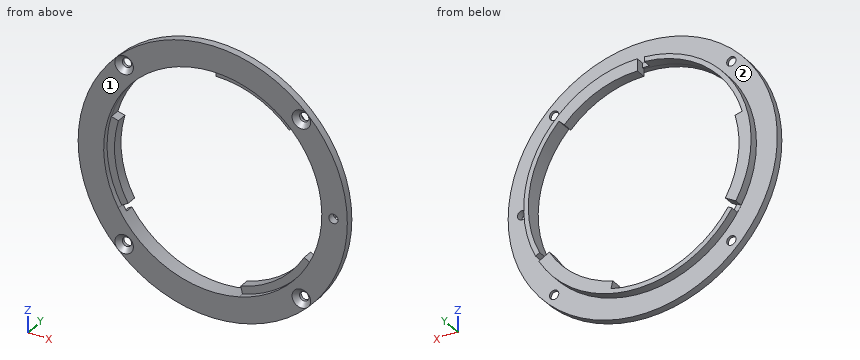
```python
from build123d import *

# Parameters (mm, degrees)
F0_R            = 29
F0_R_2          = 21.9
F1_DEPTH        = 3.5
F2_R            = 23.5
F3_DEPTH        = 1.2
F5_DEPTH        = 3.501
F6_R            = 30.5
F6_R_2          = 24.5
F7_DEPTH        = 1.9
F8_W            = 1.5
F8_H            = 25
F9_DEPTH        = 1.85
F11_D           = 2
F13_D           = 2
F13_DEPTH       = 10
F13_CSINK_D     = 4
F13_CSINK_ANGLE = 90


with BuildPart() as f1:
    # F0 (on Front) → F1 (new body)
    with BuildSketch(Plane.XZ):
        Circle(F0_R)
        Circle(F0_R_2, mode=Mode.SUBTRACT)
    extrude(amount=F1_DEPTH)

    # F2 (on face) → F3 (cut)
    with BuildSketch(Plane.XZ.offset(3.5)):
        Circle(F2_R)
    extrude(amount=-F3_DEPTH, mode=Mode.SUBTRACT)

    # F4 (on face) → F5 (cut, through all)
    with BuildSketch(Plane.XZ.offset(3.5)):
        with BuildLine():
            Line((0, 21.9), (0, 23.5))
            ThreePointArc((0, 23.5), (-14.142653, 18.767934), (-22.58965, 6.477478))
            Line((-22.58965, 6.477478), (-21.051631, 6.036458))
            ThreePointArc((-21.051631, 6.036458), (-21.736761, -2.668939), (-18.965956, -10.95))
            Line((-18.965956, -10.95), (-20.351597, -11.75))
            ThreePointArc((-20.351597, -11.75), (-9.182182, -21.631864), (5.685165, -22.80195))
            Line((5.685165, -22.80195), (5.29809, -21.249476))
            ThreePointArc((5.29809, -21.249476), (13.179749, -17.490118), (18.965956, -10.95))
            Line((18.965956, -10.95), (20.351597, -11.75))
            ThreePointArc((20.351597, -11.75), (23.324835, 2.86393), (16.904485, 16.324472))
            Line((16.904485, 16.324472), (15.753542, 15.213018))
            ThreePointArc((15.753542, 15.213018), (8.557012, 20.159056), (0, 21.9))
        make_face()
    extrude(amount=-F5_DEPTH, mode=Mode.SUBTRACT)

    # F6 (on face) → F7 (cut)
    with BuildSketch(Plane(origin=(0, 0, 0), x_dir=(-1, 0, 0), z_dir=(0, 1, 0))):
        Circle(F6_R)
        Circle(F6_R_2, mode=Mode.SUBTRACT)
    extrude(amount=-F7_DEPTH, mode=Mode.SUBTRACT)

    # F8 (on face) → F9 (cut)
    with BuildSketch(Plane(origin=(0, 0, 0), x_dir=(-1, 0, 0), z_dir=(0, 1, 0))):
        Polygon((21.650635, -12.5), (0, 0), (-0.75, -1.299038), (20.900635, -13.799038), align=None)
        with Locations((0.75, 12.5)):
            Rectangle(F8_W, F8_H)
        Polygon((-21.650635, -12.5), (0, 0), (-0.75, 1.299038), (-22.400635, -11.200962), align=None)
    extrude(amount=-F9_DEPTH, mode=Mode.SUBTRACT)

    # F11 (through all)
    with Locations(Plane.XZ.offset(3.5)):
        with Locations((26, 0)):
            Hole(F11_D / 2)

    # F13
    with Locations(Plane.XZ.offset(3.5)):
        with Locations((-19.091883, 19.091883), (19.091883, 19.091883), (19.091883, -19.091883), (-19.091883, -19.091883)):
            CounterSinkHole(F13_D / 2, F13_CSINK_D / 2, depth=F13_DEPTH, counter_sink_angle=F13_CSINK_ANGLE)


solid = f1.part
```
Work out the finished part from the listing and answer in its coordinate system (mm). Face numbers are marked on the shaded views. A direction names the side the tool comes from. Give positions to 0.01 mm unless a question says otherwise; leave off trailing zeros. Write each loop counter-clockwise with the first axis right and the second up, starting at its lowest first coordinate (ties: lowest second). Pieces come first, ordered by that corner, then holes.
(1) Straight lines are drawn through the part: line 1 (Y direction, x = -8.5, z = -24); line 2 (Z direction, x = 4.5, y = -0.6); line 3 (Z direction, x = 17, y = -1.7). For each, find the intervals that lie inside material, in ascending order.
Final values:
line 1: y = -3.5 to -1.9
line 2: z = -24.08 to -23.07, 21.43 to 24.08
line 3: z = -17.64 to -13.81, 16.22 to 17.64
(2) Flat-ended cylindrical pins translate along their axes: pin 1 Ø0.5 at (x, z) = (21, -11.5) entering from +Y; pin 2 Ø1 at (y, z) = (-0.5, -11.5) entering from +X; pin 3 Ø2.5 at (x, z) = (-21.5, -1.5) entering from -Y. Find the tip coordinate at first contact, or state that the pin passes through.
Final values:
pin 1: stops at y = -1.85
pin 2: stops at x = 20.78
pin 3: stops at y = -2.3
(3) The part is cut by section D-D on x = -15.5. Write down the section's boundary in (y, z).
Final values:
outline: (-3.5, -24.51) - (-1.9, -24.51) - (-1.9, -18.97) - (0, -18.97) - (0, -17.66) - (-3.5, -17.66) - close; (-3.5, 17.66) - (0, 17.66) - (0, 18.97) - (-1.9, 18.97) - (-1.9, 24.51) - (-3.5, 24.51) - close
(4) The part is cut by section B-B on x = 9. Write down the section's boundary in (y, z).
Final values:
outline: (-3.5, -27.57) - (-1.9, -27.57) - (-1.9, -22.79) - (0, -22.79) - (0, -19.97) - (-2.3, -19.97) - (-2.3, -21.71) - (-3.5, -21.71) - close; (-3.5, 21.71) - (-2.3, 21.71) - (-2.3, 19.97) - (0, 19.97) - (0, 22.79) - (-1.9, 22.79) - (-1.9, 27.57) - (-3.5, 27.57) - close
(5) The part is cut by section C-C on x = -6.5. Write down the section's boundary in (y, z), plus the area to 3 significant figures.
Final values:
outline: (-3.5, -28.26) - (-1.9, -28.26) - (-1.9, -23.62) - (0, -23.62) - (0, -22.58) - (-3.5, -22.58) - close; (-3.5, 22.58) - (0, 22.58) - (0, 23.62) - (-1.9, 23.62) - (-1.9, 28.26) - (-3.5, 28.26) - close
area: 22.1 mm2
(6) The part is cut by section A-A on z = 0. Write down the section's boundary in (x, y).
Final values:
outline: (-29, -3.5) - (-23.5, -3.5) - (-23.5, -2.3) - (-21.9, -2.3) - (-21.9, 0) - (-24.5, 0) - (-24.5, -1.9) - (-29, -1.9) - close; (23.5, -3.5) - (25, -3.5) - (25, -1.9) - (24.5, -1.9) - (24.5, 0) - (23.5, 0) - close; (27, -3.5) - (29, -3.5) - (29, -1.9) - (27, -1.9) - close
(7) Which of the six approach directions +Z, -Z, +X, -X, +Y, -Y give full straight-line access (tool end or side, diameter ignored) to the marked faces 1 and 2?
Final values:
face 1: +Z, -Z, +X, -X, -Y
face 2: +Y
